Verification items for this drawing (mm, ordinates from the low corner). Coordinates: 2 decimals unless noted, no trailing zeros. Write each loop counter-clockwise with the first axis right and the second up, starting at its lowest first coordinate (ties: lowest second). Pieces come first, ordered by that corner, then holes. Notation, with made-up numbers: (2, 17.25) -> (41, 17.25) arc R24 ccw to (41, 49.25) -> close; hole circle Ø7 at (30.5, -38). An arc over 180 degrees is marked (long way). One line per item, written item: value. Start each with the question number.
1) Sectioned sample at A-A on z = 14.25. Enter the section's corners in (x, y), plus the area to 4 significant figures.
2) Draft check along X on the marked faces 1, 2, 3 and 4. Enter one of: +X half, -X half, draft (parallel to the pull), parting line (faces both ways), or undercut.
3) Scan lines: line 1 along X through (y, z) = (13, 2); line 2 along Z through (x, y) = (9, 1.75). Record each from-to range of solid material in increasing order. Write a range as [from, to].
4) Sectioned sample at B-B on y = 16.75. Enter the section's corners in (x, z), plus the area to 3 significant figures.
5) Sectioned sample at C-C on x = 73. Enter the section's corners in (y, z).
6) Gauge pin test, flat end, axial feed: P1, Ø6, axis at x = 8, y = 9.5, coming from the +Z side. Record the tip position at first contact, or that the pin passes through.
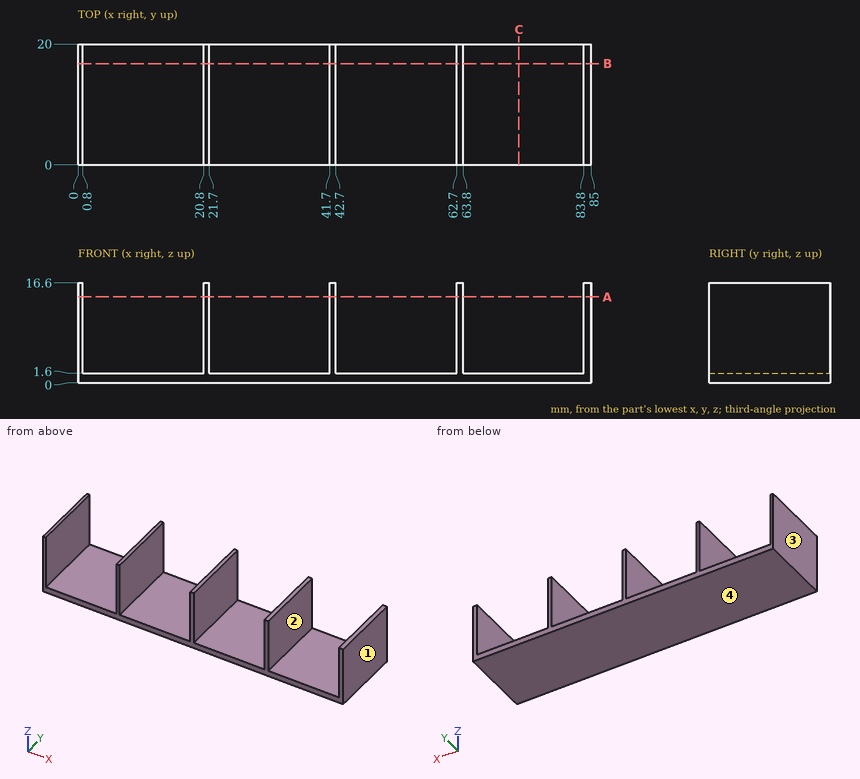
Answers:
1. outline: (0, 0) -> (0.8, 0) -> (0.8, 20) -> (0, 20) -> close; (20.8, 0) -> (21.7, 0) -> (21.7, 20) -> (20.8, 20) -> close; (41.7, 0) -> (42.7, 0) -> (42.7, 20) -> (41.7, 20) -> close; (62.7, 0) -> (63.8, 0) -> (63.8, 20) -> (62.7, 20) -> close; (83.8, 0) -> (85, 0) -> (85, 20) -> (83.8, 20) -> close
1. area: 100.0 mm2
2. face 1: +X half
2. face 2: undercut
2. face 3: -X half
2. face 4: draft
3. line 1: x = [0, 0.8], [20.8, 21.7], [41.7, 42.7], [62.7, 63.8], [83.8, 85]
3. line 2: z = [0, 1.6]
4. outline: (0, 0) -> (85, 0) -> (85, 16.6) -> (83.8, 16.6) -> (83.8, 1.6) -> (63.8, 1.6) -> (63.8, 16.6) -> (62.7, 16.6) -> (62.7, 1.6) -> (42.7, 1.6) -> (42.7, 16.6) -> (41.7, 16.6) -> (41.7, 1.6) -> (21.7, 1.6) -> (21.7, 16.6) -> (20.8, 16.6) -> (20.8, 1.6) -> (0.8, 1.6) -> (0.8, 16.6) -> (0, 16.6) -> close
4. area: 211 mm2
5. outline: (0, 0) -> (20, 0) -> (20, 1.6) -> (0, 1.6) -> close
6. P1: stops at z = 1.6
